```python
from build123d import *

# Parameters (mm, degrees)
SKETCH_3_RX         = 44.090053558
SKETCH_3_RY         = 26.443239621
EXTRUDE_1_DEPTH     = 3
CUT_EXTRUDE_START   = 3
SKETCH_3_4_RX       = 44.090053558
SKETCH_3_4_RY       = 26.443239621
SKETCH_3_4_RX_2     = 41.255952368
SKETCH_3_4_RY_2     = 22.400810242
CUT_EXTRUDE_2_DEPTH = 1


with BuildPart() as part:
    # 草图3 → 凸台-拉伸1 (new body)
    with BuildSketch(Plane.XY):
        with Locations(Location((117.824832916, 115.23790741), (0, 0, 180))):
            Ellipse(SKETCH_3_RX, SKETCH_3_RY)
    extrude(amount=EXTRUDE_1_DEPTH)

    # 草图3<4> → 切除-拉伸2 (cut)
    # profile 1 of 5: a face of its own
    with BuildSketch(Plane.XY.offset(CUT_EXTRUDE_START)):
        with Locations(Location((117.824832916, 115.23790741), (0, 0, 180))):
            Ellipse(SKETCH_3_4_RX, SKETCH_3_4_RY)
        with Locations((117.824832916, 115.23790741)):
            Ellipse(SKETCH_3_4_RX_2, SKETCH_3_4_RY_2, mode=Mode.SUBTRACT)
    # profile 2 of 5: a face of its own
    with BuildSketch(Plane.XY.offset(CUT_EXTRUDE_START)):
        with BuildLine():
            ThreePointArc((143.89906311, 119.63936615), (147.779438013, 115.207061658), (143.822433472, 110.843032837))
            Line((143.822433472, 110.843032837), (136.862030029, 110.843032837))
            Line((136.862030029, 110.843032837), (136.862030029, 106.825332642))
            Line((136.862030029, 106.825332642), (143.409423828, 106.825332642))
            ThreePointArc((143.409423828, 106.825332642), (151.457049674, 115.283053778), (143.326080322, 123.660682678))
            Line((143.326080322, 123.660682678), (132.137237549, 123.660682678))
            Line((132.137237549, 123.660682678), (132.137237549, 106.814918518))
            Line((132.137237549, 106.814918518), (136.179397583, 106.814918518))
            Line((136.179397583, 106.814918518), (136.179397583, 119.63936615))
            Line((136.179397583, 119.63936615), (142.804812511, 119.63936615))
            ThreePointArc((142.804812511, 119.63936615), (143.351937811, 119.673300221), (143.89906311, 119.63936615))
        make_face()
    # profile 3 of 5: a face of its own
    with BuildSketch(Plane.XY.offset(CUT_EXTRUDE_START)):
        with BuildLine():
            Line((124.547664698, 113.264060974), (125.282608032, 113.264060974))
            ThreePointArc((125.282608032, 113.264060974), (128.113315049, 114.623573913), (129.320327759, 117.522590637))
            Line((129.320327759, 117.522590637), (129.320327759, 123.64755249))
            Line((129.320327759, 123.64755249), (125.319236755, 123.64755249))
            Line((125.319236755, 123.64755249), (125.319236755, 117.847755432))
            ThreePointArc((125.319236755, 117.847755432), (124.968269871, 117.246162802), (124.376983643, 116.878097534))
            Line((124.376983643, 116.878097534), (116.446258545, 116.873641968))
            Line((116.446258545, 116.873641968), (116.446258545, 106.834098816))
            Line((116.446258545, 106.834098816), (120.443962097, 106.834098816))
            Line((120.443962097, 106.834098816), (120.443962097, 113.264060974))
            Line((120.443962097, 113.264060974), (124.547664698, 113.264060974))
        make_face()
    # profile 4 of 5: a face of its own
    with BuildSketch(Plane.XY.offset(CUT_EXTRUDE_START)):
        with BuildLine():
            ThreePointArc((111.588310242, 117.898681641), (111.937267918, 117.178522683), (112.678985596, 116.878097534))
            Line((112.678985596, 116.878097534), (115.696937561, 116.878097534))
            Line((115.696937561, 116.878097534), (115.696937561, 113.216255188))
            Line((115.696937561, 113.216255188), (112.02633667, 113.216255188))
            ThreePointArc((112.02633667, 113.216255188), (108.882327189, 114.5074245), (107.595947266, 117.653396606))
            Line((107.595947266, 117.653396606), (107.595947266, 123.64239502))
            Line((107.595947266, 123.64239502), (111.588310242, 123.64239502))
            Line((111.588310242, 123.64239502), (111.588310242, 117.898681641))
        make_face()
    # profile 5 of 5: a face of its own
    with BuildSketch(Plane.XY.offset(CUT_EXTRUDE_START)):
        with BuildLine():
            Line((100.320487976, 123.701698303), (85.857902527, 123.701698303))
            Line((85.857902527, 123.701698303), (85.857902527, 106.831474304))
            Line((85.857902527, 106.831474304), (89.85785675, 106.821266174))
            Line((89.85785675, 106.821266174), (89.85785675, 113.6771698))
            Line((89.85785675, 113.6771698), (99.629045068, 113.652244725))
            ThreePointArc((99.629045068, 113.652244725), (99.745733087, 113.656821169), (99.86239624, 113.651649475))
            ThreePointArc((99.86239624, 113.651649475), (101.141097708, 112.257892609), (99.86239624, 110.864135742))
            ThreePointArc((99.86239624, 110.864135742), (99.742164596, 110.858959497), (99.621932952, 110.864135742))
            Line((99.621932952, 110.864135742), (90.656356812, 110.864135742))
            Line((90.656356812, 110.864135742), (90.656356812, 106.879867554))
            Line((90.656356812, 106.879867554), (99.860228116, 106.856387052))
            Line((99.860228116, 106.856387052), (100.208221436, 106.855499268))
            ThreePointArc((100.208221436, 106.855499268), (104.731739573, 109.852213429), (104.070821683, 115.23790741))
            ThreePointArc((104.070821683, 115.23790741), (104.793856796, 120.621074732), (100.320487976, 123.701698303))
        make_face()
        with BuildLine():
            Line((89.865707397, 116.923698425), (89.865707397, 119.666885376))
            Line((89.865707397, 119.666885376), (99.797425153, 119.666885376))
            Line((99.797425153, 119.666885376), (99.823417664, 119.666885376))
            ThreePointArc((99.823417664, 119.666885376), (101.182014946, 118.28271099), (99.798248291, 116.923698425))
            Line((99.798248291, 116.923698425), (89.865707397, 116.923698425))
        make_face(mode=Mode.SUBTRACT)
    extrude(amount=-CUT_EXTRUDE_2_DEPTH, mode=Mode.SUBTRACT)


solid = part.part
```
Build history of the part. All positions in model axes, mm. A direction names the side the tool comes from. Round coordinates to 2 decimals unless told otherwise and drop trailing zeros.
1) Pin check, flat tips, straight feed: pin 1 (0.5 mm diameter, centred on x = 123.5, z = 2.5, fed in from +Y); pin 2 (0.5 mm diameter, centred on y = 121, z = 2.5, fed in from +X); pin 3 (0.5 mm diameter, centred on x = 113, z = 2.5, fed in from +Y); pin 4 (6 mm diameter, centred on x = 92.5, y = 96.5, fed in from -Z). Stop position of each tip, or through.
2) Band-saw the part on A-A, the plane z = 2.55. Give the number of separate pieces and of enclosed holes in the cut face, and give its area (3 significant figures).
3) 3-axis set-ups, long thin cutter, end or side, ignore diameter. For faces 3 (the flat face through (111, 117, 2)), 4 (the flat face through (118, 115, 0)): which of +Z, -Z, +X, -X, +Y, -Y reach the whole face in a straight line?
4) Mould opens along Y. For faces 1 (the cylindrical face through (151.456, 115.102, 2.507)), 2 (the flat face through (96, 118, 3)) say: +Y half, -Y half, draft (parallel to the pull), parting line (faces both ways), or undercut.
5) Drill centre lines: probe 1 along Y at (x, z) = (143, 2.4); probe 2 along Z at (x, y) = (97.5, 138.5); probe 3 along Y at (x, z) = (141, 2.55). Where is each one in solid material? Low to high.
Ans:
1. pin 1: stops at y = 137.44
1. pin 2: stops at x = 157.81
1. pin 3: stops at y = 137.5
1. pin 4: stops at z = 0
2. separate pieces: 2
2. enclosed holes: 4
2. area: 2,310 mm2
3. face 3: +Z
3. face 4: -Z, +X, -X, +Y, -Y
4. face 1: undercut
4. face 2: draft
5. probe 1: y = 97.49 to 106.83, 110.84 to 119.66, 123.66 to 132.98
5. probe 2: z = 0 to 2
5. probe 3: y = 96.71 to 106.83, 110.84 to 119.64, 123.66 to 133.77
